Autodesk Inventor part; units mm, degrees
ref_plane "YZ Plane" through (0, 0, 0) normal (1, 0, 0) x (0, 1, 0)
ref_plane "XZ Plane" through (0, 0, 0) normal (0, 1, 0) x (-1, 0, 0)
ref_plane "XY Plane" through (0, 0, 0) normal (0, 0, 1) x (1, 0, 0)
sketch "Sketch1" plane through (0, 0, 0) normal (1, 0, 0) x (0, 1, 0)
  line L0 (79.4172, -148.1416) -> (-70.5828, -23.1416)
  line L1 (-70.5828, -23.1416) -> (-70.5828, 26.8584)
  line L2 (-70.5828, 26.8584) -> (79.4172, 151.8584)
  line L3 (79.4172, 151.8584) -> (29.4172, 41.8584)
  line L4 (29.4172, 41.8584) -> (29.4172, -38.1416)
  line L5 (29.4172, -38.1416) -> (79.4172, -148.1416)
  line L6 (-0.5828, -43.1416) -> (-0.5828, 46.8584)
  line L7 (-0.5828, 46.8584) -> (-40.5828, 11.8584)
  line L8 (-40.5828, 11.8584) -> (-40.5828, -8.1416)
  line L9 (-40.5828, -8.1416) -> (-0.5828, -43.1416)
  point P0 (0, 0)
  dimension "d0" = 0
  dimension "d2" = 50
  dimension "d6" = 150
  dimension "d7" = 300
  dimension "d9" = 80
  dimension "d104" = 50
  dimension "d105" = 15
  dimension "d106" = 20
  dimension "d107" = 40
  dimension "d108" = 30
  dimension "d109" = 90
extrude "Extrusion2" add sketch "Sketch1" along normal blind 4
fillet "Fillet2" radius 15 2 edges at (2, 79.4172, -148.1416) (2, 79.4172, 151.8584)
hole "Hole11" at (0, 38.6064, -94.607) direction (1, 0, 0) diameter 10 end through all
hole "Hole12" at (0, 38.6064, 98.3238) direction (1, 0, 0) diameter 10 end through all
hole "Hole13" at (0, 38.6064, -94.607) direction (1, 0, 0) diameter 11.6 depth 0.8 tip angle 118
hole "Hole14" at (0, 38.6064, 98.3238) direction (1, 0, 0) diameter 11.6 depth 0.8 tip angle 118
hole "Hole15" at (4, 12.0826, 76.2206) direction (-1, 0, 0) diameter 4 depth 8
hole "Hole16" at (4, 12.0826, -72.5039) direction (-1, 0, 0) diameter 4 depth 8
hole "Hole17" at (4, -55.5828, -16.116) direction (-1, 0, 0) diameter 4 depth 8
hole "Hole18" at (4, -55.5828, 19.8328) direction (-1, 0, 0) diameter 4 depth 8
properties part number "BaseCenterPlate"
Check sheet for the modelled part. Datum: model origin and axes. Units: mm. A direction names the side the tool comes from. Round coordinates to 2 decimals unless told otherwise and drop trailing zeros. Order: outer loops, then holes, each group sorted by start corner. A loop starts at its lowest first (then second) coordinate and runs counter-clockwise, first axis right, second up.
(1) Draft check along Y on faces 4 (the flat face through (1.97, 41, 67.34)), 5 (the cylindrical face through (2, 47.9, 110.1)), 6 (the cylindrical face through (0.406, 36.864, -89.075)). Enter one of: pulls with the +Y half, pulls with the -Y half, needs draft (parallel to the pull), parting line crosses it, or undercut.
(2) Scan lines: probe 1 along Y at (x, z) = (1.75, -7); probe 2 along Z at (x, y) = (1.6, 11); probe 3 along Z at (x, y) = (1.8, -54.5). Record each from-to range of solid material in increasing order.
(3) Cross-section at C-C, the plane x = 2.9. Enter the section's corners in (y, z), and give its area (3 significant figures).
(4) Access from +Z, -Z, +X, -X, +Y, -Y to the whole of each face (thin tool, end or side, straight path). Record for faces 1 (the cylindrical face through (0.41, 38.35, 92.53)), 2 (the flat face through (1.97, 40.68, -62.92)), 3 (the flat face through (1.972, -20.303, 29.603)).
(5) Cross-section at D-D, the plane z = -60. Enter the section's corners in (x, y).
(6) Cross-section at A-A, the plane y = -12. Enter the section's corners in (x, z), and give its area (3 significant figures).
(7) Go/stop test with flat-tipped pins: P1, Ø6.5, axis at y = -55.58, z = -16.12, coming from the +X side; P2, Ø10.5, axis at y = 38.61, z = 98.32, coming from the -X side; P3, Ø2, axis at x = 1.5, z = 6, coming from the +Y side; P4, Ø8, axis at y = 38.61, z = 98.32, coming from the -X side. Record where each tip stops, or that it passes through.
(8) Cross-section at B-B, the plane z = 3. Enter the section's corners in (x, y), and give its area (3 significant figures).
Check sheet entries:
1. face 4: pulls with the +Y half
1. face 5: parting line crosses it
1. face 6: undercut
2. probe 1: y = -70.58 to -40.58, -0.58 to 29.42
2. probe 2: z = -91.13 to -74.19, -70.82 to 74.54, 77.9 to 94.84
2. probe 3: z = -36.54 to -17.8, -14.43 to 18.15, 21.51 to 40.26
3. outline: (-70.58, -23.14) - (29, -106.13) arc R15 ccw to (52.26, -88.4) - (29.42, -38.14) - (29.42, 41.86) - (52.26, 92.12) arc R15 ccw to (29, 109.85) - (-70.58, 26.86) - close; hole circle Ø4 at (-55.58, -16.12); hole circle Ø4 at (-55.58, 19.83); hole (-40.58, -8.14) - (-0.58, -43.14) - (-0.58, 46.86) - (-40.58, 11.86) - close; hole circle Ø4 at (12.08, -72.5); hole circle Ø4 at (12.08, 76.22); hole circle Ø10 at (38.61, -94.61); hole circle Ø10 at (38.61, 98.32)
3. area: 13,000 mm2
4. face 1: -X
4. face 2: +X, -X, +Y
4. face 3: +X, -X
5. outline: (0, -26.35) - (4, -26.35) - (4, 39.35) - (0, 39.35) - close
6. outline: (0, -71.96) - (4, -71.96) - (4, -33.15) - (0, -33.15) - close; (0, 36.87) - (4, 36.87) - (4, 75.68) - (0, 75.68) - close
6. area: 310 mm2
7. P1: stops at x = 4
7. P2: stops at x = 1.13
7. P3: stops at y = 29.42
7. P4: passes through
8. outline: (0, -70.58) - (4, -70.58) - (4, -40.58) - (0, -40.58) - close; (0, -0.58) - (4, -0.58) - (4, 29.42) - (0, 29.42) - close
8. area: 240 mm2
